Solid Edge part; units mm, degrees
sketch "Sketch1" plane through (0, 0, 0) normal (0, 0, 1) x (1, 0, 0)
  circle A0 centre (0, 0) radius 4
extrude "Protrusion1" add sketch "Sketch1" along normal blind 85
cosmetic_thread "Thread_1" thread depth 20
sketch "Sketch2" plane through (0, 0, 85) normal (0, 0, 1) x (1, 0, 0)
  line L0 (-3.832, 6.6372) -> (-7.664, 0)
  line L1 (-7.664, 0) -> (-3.832, -6.6372)
  line L2 (-3.832, -6.6372) -> (3.832, -6.6372)
  line L3 (3.832, -6.6372) -> (7.664, 0)
  line L4 (7.664, 0) -> (3.832, 6.6372)
  line L5 (3.832, 6.6372) -> (-3.832, 6.6372)
extrude "ExtrudedProtrusion_3" add sketch "Sketch2" along normal blind 5.6175
properties material "Steel"
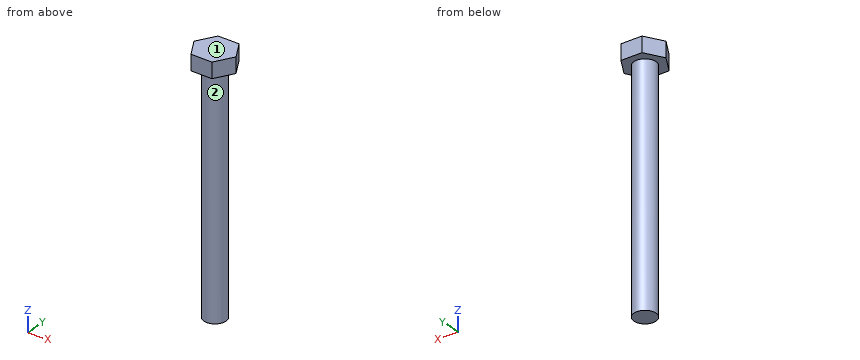
Source: CAD feature listing. Evaluate the final solid. Frame: model axes, mm. Face numbers are marked on the shaded views. A direction names the side the tool comes from. Coordinates: 2 decimals unless noted, no trailing zeros. Write each loop counter-clockwise with the first axis right and the second up, starting at its lowest first coordinate (ties: lowest second). Pieces come first, ordered by that corner, then holes. Notation, with made-up numbers: (55, -32.5) -> (83, -32.5) arc R23 ccw to (83, -22.5) -> close; hole circle Ø3 at (35.25, 29). An arc over 180 degrees is marked (long way). Return JSON: item names as keys, results as strings. Group by question number.
1) Section query B-B, the plane y = 1.5. Return loops of the section in (x, z), plus the area to 3 significant figures.
2) Section query A-A, the plane x = 0. Return loops of the section in (y, z).
3) Set-up query: the marked faces 1 and 2. Return all of +Z, -Z, +X, -X, +Y, -Y with unobstructed straight access to the full face (end or side cutting, diameter ignored); none if empty.
4) Section query C-C, the plane z = 83. Return loops of the section in (x, y), plus the area to 3 significant figures.
5) Ray query, line 1 along Z through (x, y) = (0, 5.5); line 2 along X through (y, z) = (-0.25, 30); line 3 along Y through (x, z) = (-1.5, 34). Return the intervals inside material, ascending.
6) Contact query for flat-ended pins moving along their axis: P1, Ø3, axis at x = -0.5, z = 81.5, coming from the -Y side; P2, Ø4, axis at y = 4.5, z = 39, coming from the +X side; P3, Ø5, axis at y = 4.5, z = 18.5, coming from the +X side. Output: stop coordinate, or through.
From the geometry:
{
 "1": {"outline": "(-6.8, 85) -> (-3.71, 85) -> (-3.71, 0) -> (3.71, 0) -> (3.71, 85) -> (6.8, 85) -> (6.8, 90.62) -> (-6.8, 90.62) -> close", "area": "707 mm²"},
 "2": {"outline": "(-6.64, 85) -> (-4, 85) -> (-4, 0) -> (4, 0) -> (4, 85) -> (6.64, 85) -> (6.64, 90.62) -> (-6.64, 90.62) -> close"},
 "3": {"face 1": "+Z, +X, -X, +Y, -Y", "face 2": "-Z"},
 "4": {"outline": "circle Ø8 at (0, 0)", "area": "50.3 mm²"},
 "5": {"line 1": "85 to 90.62", "line 2": "-3.99 to 3.99", "line 3": "-3.71 to 3.71"},
 "6": {"P1": "y = -4", "P2": "x = 3.12", "P3": "x = 3.46"}
}
